from build123d import *

# Parameters (mm, degrees)
BOX004_W               = 10
BOX004_H               = 10
BOX004_DEPTH           = 10
CYLINDER001_R          = 15
CYLINDER001_DEPTH      = 30
CYLINDER001_ROLL_ANGLE = 90
BOX003_W               = 8
BOX003_H               = 2
BOX003_DEPTH           = 2.5
BOX002_W               = 5
BOX002_H               = 1
BOX002_DEPTH           = 6
BOX001_W               = 5
BOX001_H               = 1
BOX001_DEPTH           = 7
CYLINDER_R             = 4
CYLINDER_DEPTH         = 2
CYLINDER_ROLL_ANGLE    = 90
BOX_W                  = 10
BOX_H                  = 20
BOX_DEPTH              = 8


with BuildPart() as obj1:
    # Box004 → Box004 (new body)
    with BuildSketch(Plane(origin=(0, 14, 0), x_dir=(1, 0, 0), z_dir=(0, 0, 1))):
        with Locations((5, 5)):
            Rectangle(BOX004_W, BOX004_H)
    extrude(amount=BOX004_DEPTH)


with BuildPart() as rounded_top:
    # Cylinder001 → Cylinder001 (new body)
    with BuildSketch(Plane.XY):
        Circle(CYLINDER001_R)
    extrude(amount=CYLINDER001_DEPTH)


with BuildPart() as rounded_top_1:
    # Cylinder001 roll: moved
    add(rounded_top.part.rotate(Axis((0, 0, 0), (1, 0, 0)), CYLINDER001_ROLL_ANGLE))


with BuildPart() as rounded_top_2:
    # Cylinder001 placement: moved
    add(rounded_top_1.part.moved(Location((5, 25, -7))))


with BuildPart() as cylinder_edge_refinement:
    # Box003 → Box003 (new body)
    with BuildSketch(Plane(origin=(1, 1, 5.5), x_dir=(1, 0, 0), z_dir=(0, 0, 1))):
        with Locations((4, 1)):
            Rectangle(BOX003_W, BOX003_H)
    extrude(amount=BOX003_DEPTH)


with BuildPart() as interior_opening:
    # Box002 → Box002 (new body)
    with BuildSketch(Plane(origin=(2.5, 3, 2), x_dir=(1, 0, 0), z_dir=(0, 0, 1))):
        with Locations((2.5, 0.5)):
            Rectangle(BOX002_W, BOX002_H)
    extrude(amount=BOX002_DEPTH)


with BuildPart() as end_opening:
    # Box001 → Box001 (new body)
    with BuildSketch(Plane(origin=(2.5, 0, 1), x_dir=(1, 0, 0), z_dir=(0, 0, 1))):
        with Locations((2.5, 0.5)):
            Rectangle(BOX001_W, BOX001_H)
    extrude(amount=BOX001_DEPTH)


with BuildPart() as solenoid_head_slot:
    # Cylinder → Cylinder (new body)
    with BuildSketch(Plane.XY):
        Circle(CYLINDER_R)
    extrude(amount=CYLINDER_DEPTH)


with BuildPart() as solenoid_head_slot_1:
    # Cylinder roll: moved
    add(solenoid_head_slot.part.rotate(Axis((0, 0, 0), (1, 0, 0)), CYLINDER_ROLL_ANGLE))


with BuildPart() as solenoid_head_slot_2:
    # Cylinder placement: moved
    add(solenoid_head_slot_1.part.moved(Location((5, 3, 5))))


with BuildPart() as cut004:
    # Box → Box (new body)
    with BuildSketch(Plane.XY):
        with Locations((5, 10)):
            Rectangle(BOX_W, BOX_H)
    extrude(amount=BOX_DEPTH)

    # Cut: cut solenoid_head_slot
    add(solenoid_head_slot_2.part, mode=Mode.SUBTRACT)

    # Cut001: cut end_opening
    add(end_opening.part, mode=Mode.SUBTRACT)

    # Cut002: cut interior_opening
    add(interior_opening.part, mode=Mode.SUBTRACT)

    # Cut003: cut cylinder_edge_refinement
    add(cylinder_edge_refinement.part, mode=Mode.SUBTRACT)

    # Common: intersect rounded_top
    add(rounded_top_2.part, mode=Mode.INTERSECT)

    # Cut004: cut obj1
    add(obj1.part, mode=Mode.SUBTRACT)


solid = cut004.part
Can you work these out from the model? Positions are in its coordinate system, mm. A direction names the side the tool comes from. Give positions to 0.01 mm unless a question says otherwise; leave off trailing zeros. Loops run counter-clockwise (first coordinate to the right, second up) from the corner with the lowest first, then second, coordinate; pieces in that order, holes last. Notation, with made-up numbers: (-7, -35.5) -> (15, -35.5) arc R23 cw to (15, -8.5) -> close; hole circle Ø10 at (-30.75, 2.5). An arc over 180 degrees is marked (long way). Use one line per item in the form item = value.
1) We'd pull the mould along Y, two halves only. Please class faces 5 (the face through (2, 1, 5)), 6 (the face through (2.5, 0.5, 4.3)), 7 (the face through (5, 14, 4)), 8 (the face through (2, 3, 4)): released by +Y, released by -Y, zero draft, split by the parting line, or undercut.
Answers:
face_5 = undercut
face_6 = zero draft
face_7 = released by +Y
face_8 = undercut
2) If we section it at C-C (x = 6.25): Please give me the cut outline in (y, z).
Answers:
outline = (0, 0) -> (14, 0) -> (14, 7.95) -> (4, 7.95) -> (4, 2) -> (3, 2) -> (3, 1.2) -> (1, 1.2) -> (1, 1) -> (0, 1) -> close
3) I need wall thicknesses on line 1 along X through (y, z) = (1.75, 5); line 2 along Y through (x, z) = (1.5, 6); line 3 along Y through (x, z) = (6, 4). Which ranges of each line are inside material? Lowest first, please.
Answers:
line_1 = 0 to 1, 9 to 10
line_2 = 0 to 1, 3 to 14
line_3 = 4 to 14
4) If we section it at B-B (z = 5): Please give me the cut outline in (x, y).
Answers:
outline = (0, 0) -> (2.5, 0) -> (2.5, 1) -> (1, 1) -> (1, 3) -> (2.5, 3) -> (2.5, 4) -> (7.5, 4) -> (7.5, 3) -> (9, 3) -> (9, 1) -> (7.5, 1) -> (7.5, 0) -> (10, 0) -> (10, 14) -> (0, 14) -> close
5) For faces 1 (the face through (10, 7, 4)), 2 (the face through (7.5, 3.5, 4.9)), 3 (the face through (5, 2, 1)), 4 (the face through (1, 2, 6)), which set-ups out of +Z, -Z, +X, -X, +Y, -Y let a thin tool reach every point of the face, with its end or its side?
Answers:
face_1 = +Z, -Z, +X, +Y, -Y
face_2 = +Z, -Y
face_3 = none
face_4 = +Z
6) If we section it at D-D (y = 11.75): Please give me the cut outline in (x, z), plus the area to 3 significant figures.
Answers:
outline = (0, 0) -> (10, 0) -> (10, 7.14) arc R15 ccw to (0, 7.14) -> close
area = 77.2 mm²
7) Will these pins go through, and if not, where does the flat tip stop? pin 1 (4 mm diameter, centred on x = 8.5, y = 5, fed in from +Z); pin 2 (0.5 mm diameter, centred on x = 4.5, y = 3.5, fed in from +Z); pin 3 (0.5 mm diameter, centred on x = 5.5, y = 0.5, fed in from +Z).
Answers:
pin_1 = 7.92
pin_2 = 2
pin_3 = 1
